Check sheet for the modelled part. Datum: model origin and axes. Units: mm. Face numbers are marked on the shaded views. A direction names the side the tool comes from. Round coordinates to 2 decimals unless told otherwise and drop trailing zeros. Loops run counter-clockwise (first coordinate to the right, second up) from the corner with the lowest first, then second, coordinate; pieces in that order, holes last. Notation, with made-up numbers: (-2, 65.25) - (13, 65.25) arc R11 cw to (13, 80.25) - close; hole circle Ø2 at (-16.5, 70). An arc over 180 degrees is marked (long way). Return JSON: item names as keys, results as strings.
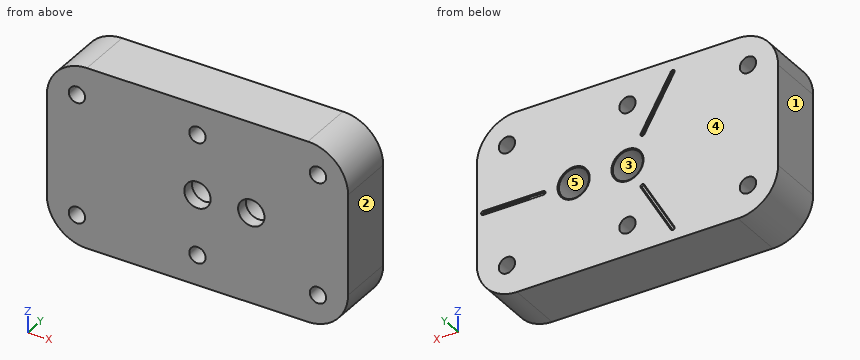
from build123d import *

# Parameters (mm, degrees)
SKETCH1_W                                   = 190.5
SKETCH1_H                                   = 114.3
EXTRUDE1_DEPTH                              = 35.56
F_3_8_CLEARANCE_HOLE1_D                     = 10.31748
LPATTERN6_COUNT                             = 3
LPATTERN6_PITCH                             = 76.2
LPATTERN6_COUNT_DIR2                        = 2
LPATTERN6_PITCH_DIR2                        = 76.2
F_5_8_11_TAPPED_HOLE1_D                     = 15.875
F_5_8_11_TAPPED_HOLE1_CSINK_D               = 17.145
F_5_8_11_TAPPED_HOLE1_CSINK_ANGLE           = 120
FILLET1_R                                   = 25.4
EXTRUDE2_DEPTH                              = 0.635
EXTRUDE2_TAPER                              = 45
TAPPED_HOLE_FOR_5_8_11_HELICOIL2_AT_2_COUNT = 2
TAPPED_HOLE_FOR_5_8_11_HELICOIL2_AT_2_PITCH = 34.036


with BuildPart() as part:
    # Sketch1 → Extrude1 (new body)
    with BuildSketch(Plane(origin=(0, 0, 0), x_dir=(1, 0, 0), z_dir=(0, 1, 0))):
        Rectangle(SKETCH1_W, SKETCH1_H)
    extrude(amount=EXTRUDE1_DEPTH)

    # 3/8 Clearance Hole1 (through all)
    with Locations(Plane(origin=(0, 35.56, 0), x_dir=(-1, 0, 0), z_dir=(0, 1, 0))):
        with Locations((76.2, -38.1)):
            f_3_8_clearance_hole1 = Hole(F_3_8_CLEARANCE_HOLE1_D / 2)

    # LPattern6: 3_8 Clearance Hole1 3 × 2
    with Locations(*[(i * LPATTERN6_PITCH, 0, j * LPATTERN6_PITCH_DIR2) for i in range(LPATTERN6_COUNT) for j in range(LPATTERN6_COUNT_DIR2) if (i, j) != (0, 0)]):
        add(f_3_8_clearance_hole1, mode=Mode.SUBTRACT)

    # 5/8-11 Tapped Hole1 (through all)
    with Locations(Plane(origin=(0, 35.56, 0), x_dir=(-1, 0, 0), z_dir=(0, 1, 0))):
        with Locations((0, 0), (-34.036, 0)):
            CounterSinkHole(F_5_8_11_TAPPED_HOLE1_D / 2, F_5_8_11_TAPPED_HOLE1_CSINK_D / 2, counter_sink_angle=F_5_8_11_TAPPED_HOLE1_CSINK_ANGLE)

    # Fillet1
    fillet1_edges = [part.edges().sort_by_distance(p)[0] for p in [
        (95.25, 17.78, 57.15),
        (-95.25, 17.78, 57.15),
        (-95.25, 17.78, -57.15),
        (95.25, 17.78, -57.15),
    ]]
    fillet(fillet1_edges, radius=FILLET1_R)

    # Sketch6 → Extrude2 (cut)
    with BuildSketch(Plane(origin=(0, 35.56, 0), x_dir=(1, 0, 0), z_dir=(0, 1, 0))):
        with BuildLine():
            Line((-8.425147737, 17.132783942), (-27.475147737, 50.128351826))
            ThreePointArc((-27.475147737, 50.128351826), (-29.21, 50.593204089), (-29.674852263, 48.858351826))
            Line((-29.674852263, 48.858351826), (-10.624852263, 15.862783942))
            ThreePointArc((-10.624852263, 15.862783942), (-8.89, 15.397931679), (-8.425147737, 17.132783942))
        make_face()
        with BuildLine():
            Line((-10.624852263, -15.862783942), (-29.674852263, -48.858351826))
            ThreePointArc((-29.674852263, -48.858351826), (-29.21, -50.593204089), (-27.475147737, -50.128351826))
            Line((-27.475147737, -50.128351826), (-8.425147737, -17.132783942))
            ThreePointArc((-8.425147737, -17.132783942), (-8.89, -15.397931679), (-10.624852263, -15.862783942))
        make_face()
        with BuildLine():
            Line((53.086, -1.27), (91.186, -1.27))
            ThreePointArc((91.186, -1.27), (92.456, 0), (91.186, 1.27))
            Line((91.186, 1.27), (53.086, 1.27))
            ThreePointArc((53.086, 1.27), (51.816, 0), (53.086, -1.27))
        make_face()
    extrude(amount=-EXTRUDE2_DEPTH, taper=EXTRUDE2_TAPER, mode=Mode.SUBTRACT)

    # Sketch9 → Tapped Hole for 5/8-11 Helicoil2 (revolve, cut)
    with BuildSketch(Plane(origin=(0, 35.56, 0), x_dir=(0, 0, 1), z_dir=(1, 0, 0))):
        Polygon((0, 0), (0, 43.056616175), (8.33374, 38.0492), (8.33374, 27.7876), (9.49579, 27.7876), (9.49579, 0.383481822), (10.16, 0), align=None)
    tapped_hole_for_5_8_11_helicoil2 = revolve(axis=Axis((0, 41.91, 0), (0, -1, 0)), mode=Mode.SUBTRACT)

    # Tapped Hole for 5/8-11 Helicoil2 at 2: Tapped Hole for 5/8-11 Helicoil2 ×2
    with Locations(*[(i * TAPPED_HOLE_FOR_5_8_11_HELICOIL2_AT_2_PITCH, 0, 0) for i in range(1, TAPPED_HOLE_FOR_5_8_11_HELICOIL2_AT_2_COUNT)]):
        add(tapped_hole_for_5_8_11_helicoil2, mode=Mode.SUBTRACT)


solid = part.part
Q1. Sectioned sample at B-B (x = 76.2). Enter the section's corners in (y, z) (3 decimals).
Answer key:
{"outline": "(0, -56.343) - (35.56, -56.343) - (35.56, -43.259) - (0, -43.259) - close; (0, -32.941) - (35.56, -32.941) - (35.56, -1.27) - (34.925, -0.635) - (34.925, 0.635) - (35.56, 1.27) - (35.56, 32.941) - (0, 32.941) - close; (0, 43.259) - (35.56, 43.259) - (35.56, 56.343) - (0, 56.343) - close"}
Q2. Sectioned sample at A-A (x = 0). Enter the section's corners in (y, z), plus the area to 3 significant figures.
Answer key:
{"outline": "(0, -57.15) - (35.56, -57.15) - (35.56, -43.26) - (0, -43.26) - close; (0, -32.94) - (35.56, -32.94) - (35.56, -10.16) - (35.18, -9.5) - (7.77, -9.5) - (7.77, -8.33) - (0, -8.33) - close; (0, 8.33) - (7.77, 8.33) - (7.77, 9.5) - (35.18, 9.5) - (35.56, 10.16) - (35.56, 32.94) - (0, 32.94) - close; (0, 43.26) - (35.56, 43.26) - (35.56, 57.15) - (0, 57.15) - close", "area": "2,670 mm²"}
Q3. Depth check by flat-ended pin: P1, Ø9.5, axis at x = 4, z = 1, coming from the +Y side; P2, Ø9.5, axis at x = 30.5, z = -3.5, coming from the +Y side; P3, Ø4, axis at x = -73.5, y = 29, coming from the +Z side. Enter the tip coordinate at first touch or a pass-through.
Answer key:
{"P1": "stops at y = 7.77", "P2": "stops at y = 35.31", "P3": "stops at z = 57.1"}
Q4. Draft check along X on the marked faces 1, 2 and 3. Enter one of: released by +X, released by -X, zero draft, split by the parting line, or undercut.
Answer key:
{"face 1": "released by -X", "face 2": "released by +X", "face 3": "undercut"}
Q5. Sectioned sample at C-C (y = 13). State how many separate pieces and enclosed holes the cut face has, plus the area to 3 significant figures.
Answer key:
{"separate pieces": "1", "enclosed holes": "8", "area": "20,200 mm²"}
Q6. Tool access check on the marked faces 4 and 5. Record the directions out of +Z, -Z, +X, -X, +Y, -Y that give a thin tool (end or side, any length) a straight path to the whole face; none if there is none.
Answer key:
{"face 4": "+Z, -Z, +X, -X, +Y", "face 5": "+Y"}
Q7. Scan lines: probe 1 along X at (y, z) = (4.5, 0); probe 2 along Z at (x, y) = (0, 25.5); probe 3 along X at (y, z) = (25.5, -4.5). Record each from-to range of solid material in increasing order. Write a range as [from, to].
Answer key:
{"probe 1": "x = [-95.25, -8.33], [8.33, 25.7], [42.37, 95.25]", "probe 2": "z = [-57.15, -43.26], [-32.94, -9.5], [9.5, 32.94], [43.26, 57.15]", "probe 3": "x = [-95.25, -8.36], [8.36, 25.67], [42.4, 95.25]"}
